from build123d import *

# Parameters (mm, degrees)
F1_DEPTH      = 11.1125
F2_R          = 3.175
F2_R_2        = 1.5875
F2_R_3        = 2.15265
F3_DEPTH      = 8.73125
F4_R          = 2.38125
F5_DEPTH      = 1.5875
F6_R          = 3.96875
F6_R_2        = 3.175
F7_DEPTH      = 2.746375
F7_DEPTH_BACK = 5.55625
F8_R          = 5.55624
F10_R         = 3.96875
F11_DEPTH     = 5.55625
F12_C1_SIZE   = 2.38125
F12_C2_SIZE   = 2.38125
F12_C3_SIZE   = 2.38125


# Not quite as in the source:
# - a fillet or chamfer is up to 0.001 mm smaller than in the source, because OpenCascade refuses the exact size


with BuildPart() as f1:
    # F0 (on Top) → F1 (new body)
    with BuildSketch(Plane.XY):
        Polygon((-12.7, 0), (0, 0), (0, -6.35), (11.1125, -6.35), (11.1125, 0), (26.9875, 0), (26.9875, -6.35), (38.1, -6.35), (38.1, -3.571875), (50.8, -3.571875), (50.8, 1.5875), (38.1, 1.5875), (38.1, 2.38125), (-12.7, 2.38125), align=None)
    extrude(amount=F1_DEPTH)

    # F2 (on face) → F3 (cut, through all)
    with BuildSketch(Plane(origin=(0, 2.38125, 0), x_dir=(-1, 0, 0), z_dir=(0, 1, 0))):
        with Locations((-45.24375, 5.55625)):
            Circle(F2_R)
        with Locations((7.14375, 5.55625)):
            Circle(F2_R_2)
        with Locations((-5.55625, 5.55625)):
            Circle(F2_R_3)
        with Locations((-32.54375, 5.55625)):
            Circle(F2_R_3)
    extrude(amount=-F3_DEPTH, mode=Mode.SUBTRACT)

    # F4 (on face) → F5 (cut)
    with BuildSketch(Plane.XZ):
        with Locations((-7.14375, 5.55625)):
            Circle(F4_R)
    extrude(amount=-F5_DEPTH, mode=Mode.SUBTRACT)

    # F6 (on face) → F7 (join, two sides)
    with BuildSketch(Plane(origin=(0, 1.5875, 0), x_dir=(-1, 0, 0), z_dir=(0, 1, 0))) as f7_sk:
        with Locations((-45.24375, 5.55625)):
            Circle(F6_R)
        with Locations((-45.24375, 5.55625)):
            Circle(F6_R_2, mode=Mode.SUBTRACT)
    extrude(amount=F7_DEPTH)
    extrude(f7_sk.sketch, amount=-F7_DEPTH_BACK)

    # F8 (radius 5.55625 in the source; OpenCascade refuses exactly that, so slightly less here)
    f8_edges = [f1.edges().sort_by_distance(p)[0] for p in [
        (0, -3.175, 0),
        (0, -3.175, 11.1125),
        (38.1, -4.960938, 0),
        (38.1, -4.960938, 11.1125),
        (38.1, 1.984375, 0),
        (38.1, 1.984375, 11.1125),
        (11.1125, -3.175, 11.1125),
        (11.1125, -3.175, 0),
        (26.9875, -3.175, 11.1125),
        (26.9875, -3.175, 0),
        (50.8, -0.992188, 11.1125),
        (50.8, -0.992188, 0),
        (-12.7, 1.190625, 11.1125),
        (-12.7, 1.190625, 0),
    ]]
    fillet(f8_edges, radius=F8_R)

    # F10 (on face) → F11 (cut, through all)
    with BuildSketch(Plane(origin=(0, 2.38125, 0), x_dir=(-1, 0, 0), z_dir=(0, 1, 0))):
        with Locations((-32.54375, 5.55625)):
            Circle(F10_R)
        with Locations((-5.55625, 5.55625)):
            Circle(F10_R)
    extrude(amount=-F11_DEPTH, mode=Mode.SUBTRACT)

    # F12: chamfer of 2.38125 on 5 edges, made by hand

    # F12_c1
    f12_c1_edges = [f1.edges().sort_by_distance(p)[0] for p in [
        (1.6273850181, 0, 9.4851149819),
        (0, 0, 5.55625),
        (1.6273850181, 0, 1.6273850181),
    ]]
    chamfer(f12_c1_edges, length=F12_C1_SIZE)

    # F12_c2
    f12_c2_edges = [f1.edges().sort_by_distance(p)[0] for p in [
        (28.6148850181, 0, 9.4851149819),
        (26.9875, 0, 5.55625),
        (28.6148850181, 0, 1.6273850181),
    ]]
    chamfer(f12_c2_edges, length=F12_C2_SIZE)

    # F12_c3
    f12_c3_edges = [f1.edges().sort_by_distance(p)[0] for p in [
        (11.1125, 0, 5.55625),
        (9.4851149819, 0, 9.4851149819),
        (9.4851149819, 0, 1.6273850181),
    ]]
    chamfer(f12_c3_edges, length=F12_C3_SIZE)


solid = f1.part
Source: CAD feature listing. Evaluate the final solid. Frame: model axes, mm. A direction names the side the tool comes from. Give positions to 0.01 mm unless a question says otherwise; leave off trailing zeros. Write each loop counter-clockwise with the first axis right and the second up, starting at its lowest first coordinate (ties: lowest second). Pieces come first, ordered by that corner, then holes. Notation, with made-up numbers: M -34,-33.75 L 24,-33.75 A6 cw 24,-29.75 Z; hole C 77.25,26.25 d6. An arc over 180 degrees is marked long. Return JSON: item names as keys, results as strings. Group by question number.
1) Pin query (flat end, axial travel): P1, Ø1.5, axis at y = -0.5, z = 3, coming from the -X side; P2, Ø3.5, axis at x = 43, z = 5.5, coming from the -Y side; P3, Ø4, axis at x = -7, z = 6.5, coming from the -Y side; P4, Ø2, axis at x = 16.5, y = -2.5, coming from the +Z side. Return the tip coordinate at first contact, or that it passes through.
2) Pull-direction query (X, two-part tool) for faces 6 (the face through (1.58, -4.39, 9.44)), 7 (the face through (44, -3.969, 9)), 8 (the face through (35.47, -0.36, 8.24)); classes: pulls with the +X half, pulls with the -X half, needs draft (parallel to the pull), parting line crosses it, or undercut.
3) Material intervals for line 1 along X through (y, z) = (-3, 4.5); line 2 along X through (y, z) = (1.5, 4.5); line 3 along X through (y, z) = (-4, 5.25), sorted ascending. Write a range as [from, to].
4) Cut plane B-B, the plane x = -3. Output: boundary loops of the cut face in (y, z), plus the area to 3 significant figures.
5) Set-up query: faces 1 (the face through (30.8, -3.175, 3.8)), 2 (the face through (48.416, 0.241, 5.696)), 3 (the face through (26.33, -1.21, 2.98)), 4 (the face through (-4.87, 0.78, 6.27)), 5 (the face through (32, -6.35, 8)). Return all of +Z, -Z, +X, -X, +Y, -Y with unobstructed straight access to the full face (end or side cutting, diameter ignored); none if empty.
Recorded:
{
 "1": {"P1": "stops at x = -12.33", "P2": "stops at y = -3.97", "P3": "stops at y = 0", "P4": "passes through"},
 "2": {"face 6": "pulls with the -X half", "face 7": "needs draft", "face 8": "undercut"},
 "3": {"line 1": "x = [0.1, 1.73], [9.38, 11.01], [27.09, 28.72], [36.37, 42.25], [48.24, 50.7]", "line 2": "x = [-12.6, -9.28], [-5.01, 1.73], [9.38, 28.72], [36.37, 42.25], [48.24, 50.7]", "line 3": "x = [0.01, 3.43], [7.69, 11.1], [27, 30.41], [34.67, 38.09]"},
 "4": {"outline": "M 0,0 L 2.38,0 L 2.38,11.11 L 0,11.11 Z", "area": "26.5 mm²"},
 "5": {"face 1": "+Y", "face 2": "+Y, -Y", "face 3": "-Z, -Y", "face 4": "-Y", "face 5": "+Z, -Z, +X, -X, -Y"}
}
